from build123d import *

# Parameters (mm, degrees)
MODEL_W         = 1.5
MODEL_H         = 6
EXTRUDE_1_DEPTH = 2


with BuildPart() as part:
    # Model → 凸台-拉伸1 (new body)
    with BuildSketch(Plane.XY):
        Polygon((785.435098254, -35.533863858), (785.435098254, -41.446863858), (786.935098254, -41.446863858), (786.935098254, -48.147363858), (785.435098254, -48.147363858), (785.466503891, -54.069864101), (206.600074702, -63.475463858), (206.600074702, -35.533863858), (351.503693607, -35.533863858), (514.281059293, -35.533863858), (677.839139625, -35.533863858), align=None)
        with Locations((350.950492985, -48.643663858)):
            Rectangle(MODEL_W, MODEL_H, mode=Mode.SUBTRACT)
        with Locations((513.951245542, -47.152263858)):
            Rectangle(MODEL_W, MODEL_H, mode=Mode.SUBTRACT)
        with Locations((677.733784151, -45.843763858)):
            Rectangle(MODEL_W, MODEL_H, mode=Mode.SUBTRACT)
        with BuildLine():
            Line((255.385635934, -40.600624691), (220.886272881, -40.391624977))
            ThreePointArc((220.886272881, -40.391624977), (218.759668454, -41.257437629), (217.86815404, -43.373396038))
            Line((217.86815404, -43.373396038), (217.797915248, -54.967639695))
            ThreePointArc((217.797915248, -54.967639695), (218.679987229, -57.11057571), (220.825776537, -57.985683696))
            Line((220.825776537, -57.985683696), (255.328350826, -57.664607948))
            ThreePointArc((255.328350826, -57.664607948), (257.425196612, -56.782610808), (258.300379439, -54.682911728))
            Line((258.300379439, -54.682911728), (258.367406995, -43.618743532))
            ThreePointArc((258.367406995, -43.618743532), (257.501594343, -41.492139105), (255.385635934, -40.600624691))
        make_face(mode=Mode.SUBTRACT)
        with BuildLine():
            Line((343.376561044, -44.133735324), (343.317446229, -53.891755741))
            ThreePointArc((343.317446229, -53.891755741), (342.442263402, -55.99145482), (340.345417617, -56.873451961))
            Line((340.345417617, -56.873451961), (309.831033894, -57.157414209))
            ThreePointArc((309.831033894, -57.157414209), (307.685244586, -56.282306223), (306.803172604, -54.139370208))
            Line((306.803172604, -54.139370208), (306.865127466, -43.912546338))
            ThreePointArc((306.865127466, -43.912546338), (307.75664188, -41.796587929), (309.883246307, -40.930775277))
            Line((309.883246307, -40.930775277), (340.394789984, -41.115616483))
            ThreePointArc((340.394789984, -41.115616483), (342.510748392, -42.007130897), (343.376561044, -44.133735324))
        make_face(mode=Mode.SUBTRACT)
        with BuildLine():
            Line((266.384844011, -40.667258713), (298.884247648, -40.864142523))
            ThreePointArc((298.884247648, -40.864142523), (301.000206057, -41.755656937), (301.866018709, -43.882261364))
            Line((301.866018709, -43.882261364), (301.803040049, -54.278082537))
            ThreePointArc((301.803040049, -54.278082537), (300.927857222, -56.377781616), (298.831011437, -57.259778757))
            Line((298.831011437, -57.259778757), (266.328582721, -57.562241451))
            ThreePointArc((266.328582721, -57.562241451), (264.182793413, -56.687133465), (263.300721432, -54.544197451))
            Line((263.300721432, -54.544197451), (263.36672517, -43.649029774))
            ThreePointArc((263.36672517, -43.649029774), (264.258239584, -41.533071365), (266.384844011, -40.667258713))
        make_face(mode=Mode.SUBTRACT)
        with BuildLine():
            Line((364.652046592, -40.643787214), (398.722200855, -40.881122213))
            ThreePointArc((398.722200855, -40.881122213), (400.837348938, -41.774557453), (401.701230373, -43.901947122))
            Line((401.701230373, -43.901947122), (401.638680431, -52.881179864))
            ThreePointArc((401.638680431, -52.881179864), (400.762583047, -54.979090054), (398.666752779, -55.860151503))
            Line((398.666752779, -55.860151503), (364.576429773, -56.178336732))
            ThreePointArc((364.576429773, -56.178336732), (363.145224808, -55.594310395), (362.557811922, -54.164492045))
            Line((362.557811922, -54.164492045), (362.638163319, -42.629806893))
            ThreePointArc((362.638163319, -42.629806893), (363.233786812, -41.219708171), (364.652046592, -40.643787214))
        make_face(mode=Mode.SUBTRACT)
        with BuildLine():
            Line((409.711176711, -40.957672161), (445.623178301, -41.207837593))
            ThreePointArc((445.623178301, -41.207837593), (447.738326383, -42.101272833), (448.602207819, -44.228662502))
            Line((448.602207819, -44.228662502), (448.544983573, -52.443375482))
            ThreePointArc((448.544983573, -52.443375482), (447.668886189, -54.541285672), (445.573055921, -55.422347121))
            Line((445.573055921, -55.422347121), (409.66496734, -55.757498635))
            ThreePointArc((409.66496734, -55.757498635), (407.519124281, -54.882420802), (406.637022827, -52.739455411))
            Line((406.637022827, -52.739455411), (406.690334064, -43.939425485))
            ThreePointArc((406.690334064, -43.939425485), (407.582817543, -41.822510116), (409.711176711, -40.957672161))
        make_face(mode=Mode.SUBTRACT)
        with BuildLine():
            Line((456.612848306, -41.284392377), (499.068785272, -41.580143304))
            ThreePointArc((499.068785272, -41.580143304), (500.478883993, -42.175766798), (501.05480495, -43.594026577))
            Line((501.05480495, -43.594026577), (500.989716833, -52.937621934))
            ThreePointArc((500.989716833, -52.937621934), (500.40565191, -54.336228727), (499.008431732, -54.923603027))
            Line((499.008431732, -54.923603027), (456.571270482, -55.319694254))
            ThreePointArc((456.571270482, -55.319694254), (454.425427423, -54.44461642), (453.543325968, -52.301651029))
            Line((453.543325968, -52.301651029), (453.592005659, -44.2661457))
            ThreePointArc((453.592005659, -44.2661457), (454.484489138, -42.149230332), (456.612848306, -41.284392377))
        make_face(mode=Mode.SUBTRACT)
        with BuildLine():
            Line((524.966262719, -40.425528272), (566.772351734, -40.716752315))
            ThreePointArc((566.772351734, -40.716752315), (568.886543297, -41.609218056), (569.751398989, -43.734853418))
            Line((569.751398989, -43.734853418), (569.712675089, -50.118674115))
            ThreePointArc((569.712675089, -50.118674115), (568.843585982, -52.229548043), (566.740674761, -53.117731028))
            Line((566.740674761, -53.117731028), (524.907725967, -53.508182781))
            ThreePointArc((524.907725967, -53.508182781), (523.476521002, -52.924156445), (522.889108116, -51.494338094))
            Line((522.889108116, -51.494338094), (522.952379447, -42.41154795))
            ThreePointArc((522.952379447, -42.41154795), (523.54800294, -41.001449229), (524.966262719, -40.425528272))
        make_face(mode=Mode.SUBTRACT)
        with BuildLine():
            Line((577.772161323, -40.793377732), (613.674023329, -41.04347253))
            ThreePointArc((613.674023329, -41.04347253), (615.788214892, -41.935938271), (616.653070584, -44.061573634))
            Line((616.653070584, -44.061573634), (616.618923292, -49.698231202))
            ThreePointArc((616.618923292, -49.698231202), (615.743769843, -51.797900808), (613.646977903, -52.679926646))
            Line((613.646977903, -52.679926646), (577.741570583, -53.015053135))
            ThreePointArc((577.741570583, -53.015053135), (575.595727525, -52.139975302), (574.71362607, -49.99700991))
            Line((574.71362607, -49.99700991), (574.751318676, -43.775131055))
            ThreePointArc((574.751318676, -43.775131055), (575.643802155, -41.658215687), (577.772161323, -40.793377732))
        make_face(mode=Mode.SUBTRACT)
        with BuildLine():
            Line((624.673832918, -41.120097947), (668.962768968, -41.42861767))
            ThreePointArc((668.962768968, -41.42861767), (670.372867689, -42.024241164), (670.948788646, -43.442500943))
            Line((670.948788646, -43.442500943), (670.901868396, -50.178044171))
            ThreePointArc((670.901868396, -50.178044171), (670.317803474, -51.576650964), (668.920583295, -52.164025264))
            Line((668.920583295, -52.164025264), (624.647873725, -52.577248753))
            ThreePointArc((624.647873725, -52.577248753), (622.502030667, -51.70217092), (621.619929212, -49.559205528))
            Line((621.619929212, -49.559205528), (621.652990271, -44.101851271))
            ThreePointArc((621.652990271, -44.101851271), (622.54547375, -41.984935902), (624.673832918, -41.120097947))
        make_face(mode=Mode.SUBTRACT)
        with BuildLine():
            Line((690.49539131, -40.869236621), (725.101155649, -41.110302716))
            ThreePointArc((725.101155649, -41.110302716), (727.216303731, -42.003737956), (728.080185166, -44.131127625))
            Line((728.080185166, -44.131127625), (728.054828945, -47.77108965))
            ThreePointArc((728.054828945, -47.77108965), (727.178731561, -49.86899984), (725.082901293, -50.750061289))
            Line((725.082901293, -50.750061289), (690.49539131, -51.072887059))
            ThreePointArc((690.49539131, -51.072887059), (689.068579953, -50.493230381), (688.476725528, -49.07143544))
            Line((688.476725528, -49.07143544), (688.481508037, -42.8552563))
            ThreePointArc((688.481508037, -42.8552563), (689.077131531, -41.445157578), (690.49539131, -40.869236621))
        make_face(mode=Mode.SUBTRACT)
        with BuildLine():
            Line((736.09497932, -41.186886435), (772.002133094, -41.437018096))
            ThreePointArc((772.002133094, -41.437018096), (774.117281177, -42.330453336), (774.981162612, -44.457843005))
            Line((774.981162612, -44.457843005), (774.961132087, -47.333285268))
            ThreePointArc((774.961132087, -47.333285268), (774.085034703, -49.431195458), (771.989204435, -50.312256907))
            Line((771.989204435, -50.312256907), (736.081115854, -50.647408421))
            ThreePointArc((736.081115854, -50.647408421), (733.935272795, -49.772330588), (733.053171341, -47.629365197))
            Line((733.053171341, -47.629365197), (733.074136673, -44.168639758))
            ThreePointArc((733.074136673, -44.168639758), (733.966620152, -42.051724389), (736.09497932, -41.186886435))
        make_face(mode=Mode.SUBTRACT)
    extrude(amount=EXTRUDE_1_DEPTH)


solid = part.part
Design review of the part built by this model. Coordinates are the model's own, in mm. Give positions to 0.01 mm unless a question says otherwise; leave off trailing zeros. Order: outer loops, then holes, each group sorted by start corner. A loop starts at its lowest first (then second) coordinate and runs counter-clockwise, first axis right, second up.
1. Add section C-C, the plane x = 278. State the section outline as (y, z) points.
Solution:
outline: (-62.32, 0) - (-57.45, 0) - (-57.45, 2) - (-62.32, 2) - close; (-40.74, 0) - (-35.53, 0) - (-35.53, 2) - (-40.74, 2) - close
2. To check wall thickness, follow L1, parallel to Y at x = 545, z = 1.8; L2, parallel to Y at x = 421.5, z = 1.8. State the ranges of each line that lie inside material, in increasing order.
Solution:
L1: y = -57.98 to -53.32, -40.57 to -35.53
L2: y = -59.98 to -55.65, -41.04 to -35.53
3. Add section B-B, the plane z = 0.8. State how many separate pieces and enclosed holes the cut face has, then the cut area to 3 significant figures.
Solution:
separate pieces: 1
enclosed holes: 14
area: 7,310 mm2
4. For pin 1 Ø0.8 at (x, z) = (351.5, 0.5) entering from -Y; pin 2 Ø0.8 at (x, z) = (786.5, 1.5) entering from +Y; pin 3 Ø1.2 at (x, z) = (786, 1.5) entering from -Y, all flat-tipped, find the tip position at first contact; note any pin that passes through.
Solution:
pin 1: stops at y = -61.13
pin 2: stops at y = -41.45
pin 3: stops at y = -54.07
5. Add section A-A, the plane x = 645. State the section outline as (y, z) points, then the cut area to 3 significant figures.
Solution:
outline: (-56.35, 0) - (-52.39, 0) - (-52.39, 2) - (-56.35, 2) - close; (-41.26, 0) - (-35.53, 0) - (-35.53, 2) - (-41.26, 2) - close
area: 19.4 mm2
